The listing builds one solid part. Answer for the finished solid, in the listing's coordinates (mm). A direction names the side the tool comes from. Coordinates: 2 decimals unless noted, no trailing zeros. Order: outer loops, then holes, each group sorted by start corner. A loop starts at its lowest first (then second) coordinate and runs counter-clockwise, first axis right, second up. Notation, with made-up numbers: (30.5, -4) -> (65.5, -4) arc R11 ccw to (65.5, 12) -> close; hole circle Ø9 at (-39, 33.25). An arc over 180 degrees is marked (long way). Answer in a Markdown table with one row per item.
```python
from build123d import *

# Parameters (mm, degrees)
F0_R     = 4
F0_R_2   = 3.4
F1_DEPTH = 600
F2_R     = 2
F3_R     = 7


with BuildPart() as f1:
    # F0 (on Top) → F1 (new body)
    with BuildSketch(Plane.XY):
        with BuildLine():
            Line((24.15, -40), (40, -40))
            Line((40, -40), (40, -24.15))
            Line((40, -24.15), (36, -24.15))
            Line((36, -24.15), (36, -27.15))
            Line((36, -27.15), (29.244802, -27.15))
            ThreePointArc((29.244802, -27.15), (26, -20), (29.244802, -12.85))
            Line((29.244802, -12.85), (36, -12.85))
            Line((36, -12.85), (36, -15.85))
            Line((36, -15.85), (40, -15.85))
            Line((40, -15.85), (40, 15.85))
            Line((40, 15.85), (36, 15.85))
            Line((36, 15.85), (36, 12.85))
            Line((36, 12.85), (29.244802, 12.85))
            ThreePointArc((29.244802, 12.85), (26, 20), (29.244802, 27.15))
            Line((29.244802, 27.15), (36, 27.15))
            Line((36, 27.15), (36, 24.15))
            Line((36, 24.15), (40, 24.15))
            Line((40, 24.15), (40, 40))
            Line((40, 40), (24.15, 40))
            Line((24.15, 40), (24.15, 36))
            Line((24.15, 36), (27.15, 36))
            Line((27.15, 36), (27.15, 29.244802))
            ThreePointArc((27.15, 29.244802), (20, 26), (12.85, 29.244802))
            Line((12.85, 29.244802), (12.85, 36))
            Line((12.85, 36), (15.85, 36))
            Line((15.85, 36), (15.85, 40))
            Line((15.85, 40), (-15.85, 40))
            Line((-15.85, 40), (-15.85, 36))
            Line((-15.85, 36), (-12.85, 36))
            Line((-12.85, 36), (-12.85, 29.244802))
            ThreePointArc((-12.85, 29.244802), (-20, 26), (-27.15, 29.244802))
            Line((-27.15, 29.244802), (-27.15, 36))
            Line((-27.15, 36), (-24.15, 36))
            Line((-24.15, 36), (-24.15, 40))
            Line((-24.15, 40), (-40, 40))
            Line((-40, 40), (-40, 24.15))
            Line((-40, 24.15), (-36, 24.15))
            Line((-36, 24.15), (-36, 27.15))
            Line((-36, 27.15), (-29.244802, 27.15))
            ThreePointArc((-29.244802, 27.15), (-26, 20), (-29.244802, 12.85))
            Line((-29.244802, 12.85), (-36, 12.85))
            Line((-36, 12.85), (-36, 15.85))
            Line((-36, 15.85), (-40, 15.85))
            Line((-40, 15.85), (-40, -15.85))
            Line((-40, -15.85), (-36, -15.85))
            Line((-36, -15.85), (-36, -12.85))
            Line((-36, -12.85), (-29.244802, -12.85))
            ThreePointArc((-29.244802, -12.85), (-26, -20), (-29.244802, -27.15))
            Line((-29.244802, -27.15), (-36, -27.15))
            Line((-36, -27.15), (-36, -24.15))
            Line((-36, -24.15), (-40, -24.15))
            Line((-40, -24.15), (-40, -40))
            Line((-40, -40), (-24.15, -40))
            Line((-24.15, -40), (-24.15, -36))
            Line((-24.15, -36), (-27.15, -36))
            Line((-27.15, -36), (-27.15, -29.244802))
            ThreePointArc((-27.15, -29.244802), (-20, -26), (-12.85, -29.244802))
            Line((-12.85, -29.244802), (-12.85, -36))
            Line((-12.85, -36), (-15.85, -36))
            Line((-15.85, -36), (-15.85, -40))
            Line((-15.85, -40), (15.85, -40))
            Line((15.85, -40), (15.85, -36))
            Line((15.85, -36), (12.85, -36))
            Line((12.85, -36), (12.85, -29.244802))
            ThreePointArc((12.85, -29.244802), (20, -26), (27.15, -29.244802))
            Line((27.15, -29.244802), (27.15, -36))
            Line((27.15, -36), (24.15, -36))
            Line((24.15, -36), (24.15, -40))
        make_face()
        with Locations((-33.5, -33.5)):
            Circle(F0_R, mode=Mode.SUBTRACT)
        with Locations((-20, -20)):
            Circle(F0_R_2, mode=Mode.SUBTRACT)
        with Locations((33.5, -33.5)):
            Circle(F0_R, mode=Mode.SUBTRACT)
        with Locations((20, -20)):
            Circle(F0_R_2, mode=Mode.SUBTRACT)
        with Locations((-33.5, 33.5)):
            Circle(F0_R, mode=Mode.SUBTRACT)
        with Locations((-20, 20)):
            Circle(F0_R_2, mode=Mode.SUBTRACT)
        Polygon((-10, 29.5), (-10, 35), (0, 35), (10, 35), (10, 29.5), (15, 23.5), (15, 17.5), (17.5, 15), (23.5, 15), (29.5, 10), (35, 10), (35, 0), (35, -10), (29.5, -10), (23.5, -15), (17.5, -15), (15, -17.5), (15, -23.5), (10, -29.5), (10, -35), (0, -35), (-10, -35), (-10, -29.5), (-15, -23.5), (-15, -17.5), (-17.5, -15), (-23.5, -15), (-29.5, -10), (-35, -10), (-35, 0), (-35, 10), (-29.5, 10), (-23.5, 15), (-17.5, 15), (-15, 17.5), (-15, 23.5), align=None, mode=Mode.SUBTRACT)
        with Locations((20, 20)):
            Circle(F0_R_2, mode=Mode.SUBTRACT)
        with Locations((33.5, 33.5)):
            Circle(F0_R, mode=Mode.SUBTRACT)
    extrude(amount=F1_DEPTH)

    # F2
    f2_edges = [f1.edges().sort_by_distance(p)[0] for p in [
        (-10, 35, 300),
        (10, 35, 300),
        (35, 10, 300),
        (35, -10, 300),
        (-35, 10, 300),
        (-35, -10, 300),
        (10, -35, 300),
        (-10, -35, 300),
    ]]
    fillet(f2_edges, radius=F2_R)

    # F3
    f3_edges = [f1.edges().sort_by_distance(p)[0] for p in [
        (-15, 23.5, 300),
        (15, 23.5, 300),
        (23.5, 15, 300),
        (-23.5, 15, 300),
        (-23.5, -15, 300),
        (23.5, -15, 300),
        (15, -23.5, 300),
        (-15, -23.5, 300),
    ]]
    fillet(f3_edges, radius=F3_R)


solid = f1.part
```
(1) Which of the six approach directions +Z, -Z, +X, -X, +Y, -Y give full straight-line access (tool end or side, diameter ignored) to faces 5 (the flat face through (-40, 32, 296)), 6 (the cylindrical face through (20, -26, 296))?
Check values:
| item | result |
|---|---|
| face 5 | +Z, -Z, -X, +Y, -Y |
| face 6 | +Z, -Z |
(2) Flat-ended cylindrical pins translate along their axes: pin 1 (1 mm diameter, centred on x = 19, z = 150.5, fed in from +Y); pin 2 (3 mm diameter, centred on y = 19.5, z = 442, fed in from +X); pin 3 (3 mm diameter, centred on y = 22, z = 438.5, fed in from -X). Find the tip coordinate at first contact, or state that the pin passes through.
Check values:
| item | result |
|---|---|
| pin 1 | y = 26.12 |
| pin 2 | x = 26.21 |
| pin 3 | x = -26.67 |
(3) A cutting plane is placed at A-A, the plane x = -1. Determine the outline of the cut face in (y, z).
Check values:
| item | result |
|---|---|
| outline | (-40, 0) -> (-35, 0) -> (-35, 600) -> (-40, 600) -> close; (35, 0) -> (40, 0) -> (40, 600) -> (35, 600) -> close |
(4) Find the intervals of material crossed by line 1 along X through (y, z) = (19.5, 510.5); line 2 along Y through (x, z) = (-20, 184); line 3 along Y through (x, z) = (-33.5, 454), in increasing order. Write a range as from..to.
Check values:
| item | result |
|---|---|
| line 1 | -26.01..-23.36, -16.64..-15, 15..16.64, 23.36..26.01 |
| line 2 | -26..-23.4, -16.6..-15, 15..16.6, 23.4..26 |
| line 3 | -40..-37.5, -29.5..-27.15, -12.85..-9.94, 9.94..12.85, 27.15..29.5, 37.5..40 |
(5) A cutting plane is placed at B-B, the plane z = 471. Count the separate pieces of the cut face and the enclosed holes in it, then the cut area to 3 significant figures.
Check values:
| item | result |
|---|---|
| separate pieces | 1 |
| enclosed holes | 9 |
| area | 1,800 mm² |
(6) For a pull along Y with two mould halves and no side action, classify faces 1 (the flat face through (0, -40, 296)), 2 (the cylindrical face through (-26, 20, 296)), 3 (the flat face through (40, 0, 296)), 4 (the flat face through (35, 0, 296)) as released by +Y, released by -Y, zero draft, split by the parting line, or undercut.
Check values:
| item | result |
|---|---|
| face 1 | released by -Y |
| face 2 | undercut |
| face 3 | zero draft |
| face 4 | undercut |
